Part model, mm, in its own coordinate system. A direction names the side the tool comes from. Give positions to 0.01 mm unless a question says otherwise; leave off trailing zeros. Write each loop counter-clockwise with the first axis right and the second up, starting at its lowest first coordinate (ties: lowest second). Pieces come first, ordered by that corner, then holes. Notation, with made-up numbers: M 68.25,-13.5 L 90.25,-13.5 A19 ccw 90.25,6.5 Z; hole C -1.5,25.5 d5. An arc over 180 degrees is marked long. Use a Markdown table: item, result.
```python
from build123d import *

# Parameters (mm, degrees)
SKETCH2_W                = 2.5
SKETCH2_H                = 2.5
SKETCH2_W_2              = 14.143059905
SKETCH2_H_2              = 13
SKETCH2_W_3              = 3
SKETCH2_H_3              = 7
BOSS_EXTRUDE1_DEPTH      = 40
SKETCH3_R                = 2.05
CUT_EXTRUDE2_DEPTH       = 40
BOSS_EXTRUDE11_DEPTH     = 30
SKETCH16_R               = 1.25
CUT_EXTRUDE9_DEPTH       = 3.5
SKETCH17_R               = 1.25
CUT_EXTRUDE10_DEPTH      = 3.5
SKETCH18_W               = 19.143059905
SKETCH18_H               = 3
BOSS_EXTRUDE4_DEPTH      = 15.5
BOSS_EXTRUDE5_DEPTH      = 13
BOSS_EXTRUDE5_DEPTH_BACK = 2
SKETCH19_W               = 19.143059905
SKETCH19_H               = 3
BOSS_EXTRUDE6_DEPTH      = 2.5
BOSS_EXTRUDE8_DEPTH      = 2.5
BOSS_EXTRUDE9_DEPTH      = 2.5
BOSS_EXTRUDE10_DEPTH     = 2.5
SKETCH25_R               = 2.05
CUT_EXTRUDE12_DEPTH      = 3.5
SKETCH27_W               = 6.543059905
SKETCH27_H               = 2.5
BOSS_EXTRUDE12_DEPTH     = 12
FILLET1_R                = 1
CUT_EXTRUDE13_DEPTH      = 78.840525416
CUT_EXTRUDE14_DEPTH      = 78.280272448


with BuildPart() as part:
    # Sketch2 → Boss-Extrude1 (new body)
    with BuildSketch(Plane(origin=(0, 0, 0), x_dir=(1, 0, 0), z_dir=(0, 1, 0))):
        with Locations((-12.826483829, 1.092750264)):
            Rectangle(SKETCH2_W, SKETCH2_H)
        with Locations((-4.504953877, 1.092750264)):
            Rectangle(SKETCH2_W_2, SKETCH2_H)
        with Locations((-12.826483829, -6.657249736)):
            Rectangle(SKETCH2_W, SKETCH2_H_2)
        with Locations((3.816576076, 1.092750264)):
            Rectangle(SKETCH2_W, SKETCH2_H)
        Polygon((-11.576483829, -13.157249736), (-14.076483829, -13.157249736), (-14.076483829, -15.657249736), (-10.776483829, -15.657249736), (-7.776483829, -15.657249736), (-7.776483829, -13.157249736), align=None)
        with Locations((3.816576076, -6.657249736)):
            Rectangle(SKETCH2_W, SKETCH2_H_2)
        Polygon((5.066576076, -13.157249736), (2.566576076, -13.157249736), (-1.233423924, -13.157249736), (-1.233423924, -15.657249736), (1.766576076, -15.657249736), (5.066576076, -15.657249736), align=None)
        with Locations((-9.276483829, -19.157249736)):
            Rectangle(SKETCH2_W_3, SKETCH2_H_3)
        with Locations((0.266576076, -19.157249736)):
            Rectangle(SKETCH2_W_3, SKETCH2_H_3)
    extrude(amount=BOSS_EXTRUDE1_DEPTH)

    # Sketch3 → Cut-Extrude2 (cut)
    with BuildSketch(Plane.ZY.offset(10.776483829)):
        with Locations((19.157249736, 30)):
            Circle(SKETCH3_R)
        with Locations((19.157249736, 7)):
            Circle(SKETCH3_R)
    extrude(amount=-CUT_EXTRUDE2_DEPTH, mode=Mode.SUBTRACT)

    # Sketch26 → Boss-Extrude11 (add)
    with BuildSketch(Plane(origin=(0, 40, 0), x_dir=(1, 0, 0), z_dir=(0, 1, 0))):
        Polygon((-1.233423924, -15.657249736), (1.766576076, -15.657249736), (5.066576076, -15.657249736), (5.066576076, 2.342750264), (-14.076483829, 2.342750264), (-14.076483829, -15.657249736), (-7.776483829, -15.657249736), (-7.776483829, -13.157249736), (-11.576483829, -13.157249736), (-11.576483829, -0.157249736), (2.566576076, -0.157249736), (2.566576076, -13.157249736), (-1.233423924, -13.157249736), align=None)
    extrude(amount=BOSS_EXTRUDE11_DEPTH)

    # Sketch16 → Cut-Extrude9 (cut)
    with BuildSketch(Plane.XY.offset(15.657249736)):
        with Locations((-9.776483829, 50)):
            Circle(SKETCH16_R)
    extrude(amount=-CUT_EXTRUDE9_DEPTH, mode=Mode.SUBTRACT)

    # Sketch17 → Cut-Extrude10 (cut)
    with BuildSketch(Plane.XY.offset(15.657249736)):
        with Locations((0.766576076, 50)):
            Circle(SKETCH17_R)
    extrude(amount=-CUT_EXTRUDE10_DEPTH, mode=Mode.SUBTRACT)

    # Sketch18 → Boss-Extrude4 (add)
    with BuildSketch(Plane(origin=(0, 0, 13.157249736), x_dir=(-1, 0, 0), z_dir=(0, 0, -1))):
        with Locations((4.504953877, 68.5)):
            Rectangle(SKETCH18_W, SKETCH18_H)
    extrude(amount=-BOSS_EXTRUDE4_DEPTH)

    # Sketch19 → Boss-Extrude5 (add, two sides: drawn at the far end of the back side and taken through both)
    with BuildSketch(Plane(origin=(0, 0, -2.342750264), x_dir=(-1, 0, 0), z_dir=(0, 0, -1)).offset(-BOSS_EXTRUDE5_DEPTH_BACK)):
        with Locations((4.504953877, 68.5)):
            Rectangle(SKETCH19_W, SKETCH19_H)
    extrude(amount=BOSS_EXTRUDE5_DEPTH + BOSS_EXTRUDE5_DEPTH_BACK)

    # Sketch21 → Boss-Extrude6 (add)
    with BuildSketch(Plane.ZY.offset(14.076483829)):
        Polygon((28.657249736, 67), (15.657249736, 53), (15.657249736, 67), align=None)
    extrude(amount=-BOSS_EXTRUDE6_DEPTH)

    # Sketch22 → Boss-Extrude8 (add)
    with BuildSketch(Plane(origin=(5.066576076, 0, 0), x_dir=(0, 0, -1), z_dir=(1, 0, 0))):
        Polygon((-28.657249736, 67), (-15.657249736, 67), (-15.657249736, 53), align=None)
    extrude(amount=-BOSS_EXTRUDE8_DEPTH)

    # Sketch23 → Boss-Extrude9 (add)
    with BuildSketch(Plane(origin=(5.066576076, 0, 0), x_dir=(0, 0, -1), z_dir=(1, 0, 0))):
        Polygon((-13.157249736, 70), (-13.157249736, 53), (15.342750264, 67), (15.342750264, 70), align=None)
    extrude(amount=-BOSS_EXTRUDE9_DEPTH)

    # Sketch24 → Boss-Extrude10 (add)
    with BuildSketch(Plane.ZY.offset(14.076483829)):
        Polygon((13.157249736, 70), (-15.342750264, 70), (-15.342750264, 67), (13.157249736, 53), align=None)
    extrude(amount=-BOSS_EXTRUDE10_DEPTH)

    # Sketch25 → Cut-Extrude12 (cut)
    with BuildSketch(Plane(origin=(0, 70, 0), x_dir=(1, 0, 0), z_dir=(0, 1, 0))):
        with Locations(Location((-4.704953829, 8.842750264, 0), (0, 0, 270))):
            Circle(SKETCH25_R)
        with Locations(Location((-4.504953767, -22.157249736, 0), (0, 0, 270))):
            Circle(SKETCH25_R)
    extrude(amount=-CUT_EXTRUDE12_DEPTH, mode=Mode.SUBTRACT)

    # Sketch27 → Boss-Extrude12 (add)
    with BuildSketch(Plane.XZ.offset(-67)):
        with Locations((-4.504953877, 14.407249736)):
            Rectangle(SKETCH27_W, SKETCH27_H)
    extrude(amount=BOSS_EXTRUDE12_DEPTH)

    # Fillet1
    fillet1_edges = [part.edges().sort_by_distance(p)[0] for p in [
        (-1.233423924, 55, 14.407249736),
        (-7.776483829, 55, 14.407249736),
    ]]
    fillet(fillet1_edges, radius=FILLET1_R)

    # Sketch28 → Cut-Extrude13 (cut, through all)
    with BuildSketch(Plane.XY.offset(15.657249736)):
        Polygon((-3.621040447, 66.996521667), (-6.803020962, 63.814541152), (-5.3888074, 62.40032759), (-2.206826885, 65.582308105), align=None)
        Polygon((-3.621040447, 63.496521667), (-6.803020962, 60.314541152), (-5.3888074, 58.90032759), (-2.206826885, 62.082308105), align=None)
        Polygon((-3.621040447, 59.996521667), (-6.803020962, 56.814541152), (-5.3888074, 55.40032759), (-2.206826885, 58.582308105), align=None)
    extrude(amount=-CUT_EXTRUDE13_DEPTH, mode=Mode.SUBTRACT)

    # Sketch29 → Cut-Extrude14 (cut, through all)
    with BuildSketch(Plane(origin=(1.766576076, 0, 0), x_dir=(0, 0, -1), z_dir=(1, 0, 0))):
        Polygon((-15.657249736, 40), (-22.657249736, 40), (-22.657249736, 33), align=None)
    extrude(amount=-CUT_EXTRUDE14_DEPTH, mode=Mode.SUBTRACT)


solid = part.part
```
1. Cut at D-D, the plane z = 18. State how many separate pieces and enclosed holes the cut face has, then the cut area to 3 significant figures.
Findings below:
| item | result |
|---|---|
| separate pieces | 7 |
| enclosed holes | 0 |
| area | 300 mm2 |
2. Drop flat-ended pins along their axis: P1, Ø2.5, axis at y = 30, z = 19.16, coming from the +X side; P2, Ø5, axis at x = -10.5, z = -8.5, coming from the -Y side; P3, Ø1.5, axis at x = -4.5, y = 33.5, coming from the +Z side; P4, Ø5.5, axis at x = -6.5, y = 34.5, coming from the -Z side. Give the stop position or say it passes through.
Findings below:
| item | result |
|---|---|
| P1 | through |
| P2 | y = 62.53 |
| P3 | z = 0.16 |
| P4 | z = -2.34 |
3. Cut at B-B, the plane z = -7.5. Give the cut face in (x, y), then the cut area to 3 significant figures.
Findings below:
| item | result |
|---|---|
| outline | M -14.08,63.15 L -11.58,63.15 L -11.58,67 L -6.25,67 L -6.25,70 L -14.08,70 Z; M -3.16,67 L 2.57,67 L 2.57,63.15 L 5.07,63.15 L 5.07,70 L -3.16,70 Z |
| area | 67.4 mm2 |
4. Two-plate mould, pull along Y, no slides. Class faces 1 (the flat face through (-6.11, 63.12, -1.08)), 2 (the flat face through (-5, 55, 14)), 3 (the flat face through (-5, 35, 0.157)): released by +Y, released by -Y, zero draft, split by the parting line, or undercut.
Findings below:
| item | result |
|---|---|
| face 1 | undercut |
| face 2 | released by -Y |
| face 3 | zero draft |
5. Cut at A-A, the plane y = 50. Give the cut face in (x, z), then the cut area to 3 significant figures.
Findings below:
| item | result |
|---|---|
| outline | M -14.08,-2.34 L 5.07,-2.34 L 5.07,15.66 L 2.02,15.66 L 2.02,13.16 L 2.57,13.16 L 2.57,0.16 L -11.58,0.16 L -11.58,13.16 L -11.03,13.16 L -11.03,15.66 L -14.08,15.66 Z; M -8.53,13.16 L -7.78,13.16 L -7.78,15.66 L -8.53,15.66 Z; M -1.23,13.16 L -0.48,13.16 L -0.48,15.66 L -1.23,15.66 Z |
| area | 132 mm2 |
6. Tool access for faces 4 (the flat face through (2.567, 65, -7)), 5 (the flat face through (-9, 16, 22.657)), 6 (the flat face through (2.567, 62, 21)), 7 (the flat face through (-3.82, 56.97, -1.08)), 8 (the flat face through (2.567, 35, 7)): list every direction of +Z, -Z, +X, -X, +Y, -Y with a clear straight run to the whole face (end or side of a thin tool).
Findings below:
| item | result |
|---|---|
| face 4 | -Z, -Y |
| face 5 | +Z, +X, -X, -Y |
| face 6 | +Z, -Y |
| face 7 | +Z, -Z |
| face 8 | +Y, -Y |
7. Cut at C-C, the plane y = 42. Give the cut face in (x, z), then the cut area to 3 significant figures.
Findings below:
| item | result |
|---|---|
| outline | M -14.08,-2.34 L 5.07,-2.34 L 5.07,15.66 L -1.23,15.66 L -1.23,13.16 L 2.57,13.16 L 2.57,0.16 L -11.58,0.16 L -11.58,13.16 L -7.78,13.16 L -7.78,15.66 L -14.08,15.66 Z |
| area | 144 mm2 |
8. Drill centre lines: L1, parallel to Z at x = 0.5, y = 11.5; L2, parallel to X at y = 49.5, z = 1; L3, parallel to Z at x = 2, y = 56.5. Where is each one in solid material? Low to high.
Findings below:
| item | result |
|---|---|
| L1 | -2.34 to 0.16, 13.16 to 22.66 |
| L2 | -14.08 to -11.58, 2.57 to 5.07 |
| L3 | -2.34 to 0.16, 13.16 to 15.66 |
